Build history of the part. All positions in model axes, mm. A direction names the side the tool comes from. Give positions to 0.01 mm unless a question says otherwise; leave off trailing zeros. Order: outer loops, then holes, each group sorted by start corner. A loop starts at its lowest first (then second) coordinate and runs counter-clockwise, first axis right, second up. Notation, with made-up numbers: (45, -31) - (76, -31) arc R8 cw to (76, -25) - close; hole circle Ø10 at (42, 2.5). An arc over 180 degrees is marked (long way). Answer in a Markdown table with one row per item.
```python
from build123d import *

# Parameters (mm, degrees)
SKETCH1_R           = 5.6
BOSS_EXTRUDE1_DEPTH = 9
SKETCH2_R           = 3
BOSS_EXTRUDE2_DEPTH = 3.5
CHAMFER1_SIZE       = 5
CHAMFER1_SIZE2      = 1.339745962


with BuildPart() as part:
    # Sketch1 → Boss-Extrude1 (new body)
    with BuildSketch(Plane.XY):
        Circle(SKETCH1_R)
    extrude(amount=BOSS_EXTRUDE1_DEPTH)

    # Sketch2 → Boss-Extrude2 (add)
    with BuildSketch(Plane.XY.offset(9)):
        Circle(SKETCH2_R)
        with BuildLine():
            Line((-1.322875656, -1.5), (1.322875656, -1.5))
            ThreePointArc((1.322875656, -1.5), (2, 0), (1.322875656, 1.5))
            Line((1.322875656, 1.5), (-1.322875656, 1.5))
            ThreePointArc((-1.322875656, 1.5), (-2, 0), (-1.322875656, -1.5))
        make_face(mode=Mode.SUBTRACT)
    extrude(amount=BOSS_EXTRUDE2_DEPTH)

    # Chamfer1
    chamfer1_edges = [part.edges().sort_by_distance(p)[0] for p in [
        (-5.6, 0, 9),
    ]]
    chamfer1_side = [part.faces().sort_by_distance(p)[0] for p in [
        (-5.6, 0, 4.5),
    ]]
    chamfer(chamfer1_edges, length=CHAMFER1_SIZE, length2=CHAMFER1_SIZE2, reference=chamfer1_side[0])

    # Fillet1: read off the stored shape, not the designer's step
    # Fillet1 outline → Fillet1 (revolve, cut)
    with BuildSketch(Plane.XZ):
        with BuildLine():
            Line((4.652186603, 7.537287752), (4.652186603, 9))
            Line((4.652186603, 9), (3, 9))
            ThreePointArc((3, 9), (4.04607373, 8.517119759), (4.652186603, 7.537287752))
        make_face()
    revolve(axis=Axis((0, 0, 0), (0, 0, 1)), mode=Mode.SUBTRACT)


solid = part.part
```
1. Cut at A-A on y = 0. Write the cut outline in (x, z), and give its area (3 significant figures).
Check result:
| item | result |
|---|---|
| outline | (-5.6, 0) - (5.6, 0) - (5.6, 4) - (4.65, 7.54) arc R2 ccw to (3, 9) - (3, 12.5) - (2, 12.5) - (2, 9) - (-2, 9) - (-2, 12.5) - (-3, 12.5) - (-3, 9) arc R2 ccw to (-4.65, 7.54) - (-5.6, 4) - close |
| area | 100 mm² |
2. Cut at D-D on z = 2.25. Write the cut outline in (x, y).
Check result:
| item | result |
|---|---|
| outline | circle Ø11.2 at (0, 0) |
3. Drop flat-ended pins along their axis: P1, Ø1.5, axis at x = 4, z = 5.5, coming from the +Y side; P2, Ø2.5, axis at x = 0.5, y = 0, coming from the +Z side; P3, Ø5, axis at y = 3.5, z = 9, coming from the +X side. Give the stop position or say it passes through.
Check result:
| item | result |
|---|---|
| P1 | stops at y = 4.11 |
| P2 | stops at z = 9 |
| P3 | stops at x = 4.42 |
4. Which spindle directions (+Z, -Z, +X, -X, +Y, -Y) get a long thin tool onto all of the face, cutting with end or side? Do faces 4 (the face through (2, 0, 11)), 5 (the face through (0, -2, 12.5)). Say none if no direction does.
Check result:
| item | result |
|---|---|
| face 4 | +Z |
| face 5 | +Z, +X, -X, +Y, -Y |
5. Cut at C-C on x = 0. Write the cut outline in (y, z).
Check result:
| item | result |
|---|---|
| outline | (-5.6, 0) - (5.6, 0) - (5.6, 4) - (4.65, 7.54) arc R2 ccw to (3, 9) - (3, 12.5) - (1.5, 12.5) - (1.5, 9) - (-1.5, 9) - (-1.5, 12.5) - (-3, 12.5) - (-3, 9) arc R2 ccw to (-4.65, 7.54) - (-5.6, 4) - close |
6. Probe line 1 (Y direction, x = 0.5, z = 10.75); line 2 (Z direction, x = 0.25, y = -1); line 3 (X direction, y = -1, z = 11.25). List the from-to ranges inside material, lowest first.
Check result:
| item | result |
|---|---|
| line 1 | y = -2.96 to -1.5, 1.5 to 2.96 |
| line 2 | z = 0 to 9 |
| line 3 | x = -2.83 to -1.73, 1.73 to 2.83 |
7. Cut at B-B on z = 9.5. Write the cut outline in (x, y), and give its area (3 significant figures).
Check result:
| item | result |
|---|---|
| outline | circle Ø6 at (0, 0); hole (-1.32, -1.5) - (1.32, -1.5) arc R2 ccw to (1.32, 1.5) - (-1.32, 1.5) arc R2 ccw to start |
| area | 17.5 mm² |
8. Two-plate mould, pull along X, no slides. Class faces 1 (the face through (0, 1.5, 11)), 2 (the face through (-5.595, 0.246, 1.972)), 3 (the face through (0, 0, 0)): +X half, -X half, draft (parallel to the pull), parting line (faces both ways), or undercut.
Check result:
| item | result |
|---|---|
| face 1 | undercut |
| face 2 | parting line |
| face 3 | draft |
